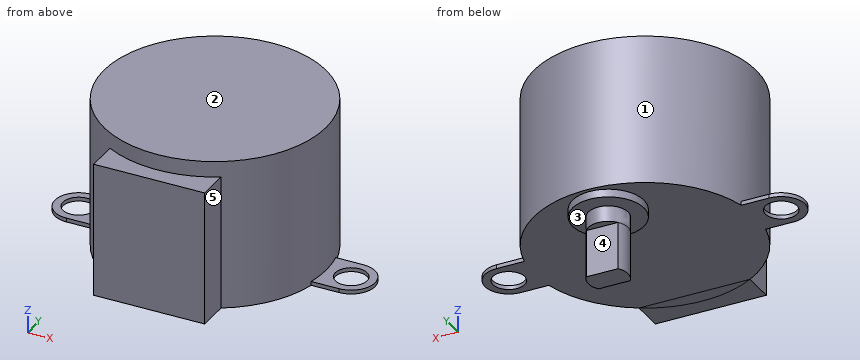
from build123d import *
from build123d.topology import SkipClean

# Parameters (mm, degrees)
SKETCH1_R           = 14
BOSS_EXTRUDE1_DEPTH = 19
SKETCH2_R           = 2
BOSS_EXTRUDE2_DEPTH = 0.5
SKETCH3_R           = 4.5
BOSS_EXTRUDE3_DEPTH = 1
SKETCH4_R           = 2.5
BOSS_EXTRUDE4_DEPTH = 2
BOSS_EXTRUDE5_DEPTH = 6
SKETCH6_W           = 14
SKETCH6_H           = 4
BOSS_EXTRUDE6_DEPTH = 17


with BuildPart() as part:
    # Sketch1 → Boss-Extrude1 (new body)
    with BuildSketch(Plane.XY):
        Circle(SKETCH1_R)
    extrude(amount=BOSS_EXTRUDE1_DEPTH)

    # Sketch2 → Boss-Extrude2 (add)
    # profile 1 of 2: a face of its own
    with BuildSketch(Plane(origin=(0, 0, 0), x_dir=(-1, 0, 0), z_dir=(0, 0, -1))):
        with BuildLine():
            Line((17.174794331, 3), (13.674794331, 3))
            ThreePointArc((13.674794331, 3), (14, 0), (13.674794331, -3))
            Line((13.674794331, -3), (17.174794331, -3))
            ThreePointArc((17.174794331, -3), (20.174794331, 0), (17.174794331, 3))
        make_face()
        with Locations((17.174794331, 0)):
            Circle(SKETCH2_R, mode=Mode.SUBTRACT)
    # profile 2 of 2: a face of its own
    with BuildSketch(Plane(origin=(0, 0, 0), x_dir=(-1, 0, 0), z_dir=(0, 0, -1))):
        with BuildLine():
            Line((-17.174794331, -3), (-13.674794331, -3))
            ThreePointArc((-13.674794331, -3), (-14, 0), (-13.674794331, 3))
            Line((-13.674794331, 3), (-17.174794331, 3))
            ThreePointArc((-17.174794331, 3), (-20.174794331, 0), (-17.174794331, -3))
        make_face()
        with Locations(Location((-17.174794331, 0, 0), (0, 0, 180))):
            Circle(SKETCH2_R, mode=Mode.SUBTRACT)
    extrude(amount=-BOSS_EXTRUDE2_DEPTH)

    # Sketch3 → Boss-Extrude3 (add)
    with BuildSketch(Plane(origin=(0, 0, 0), x_dir=(-1, 0, 0), z_dir=(0, 0, -1))):
        with Locations(Location((0, 9, 0), (0, 0, 180))):
            Circle(SKETCH3_R)
    extrude(amount=BOSS_EXTRUDE3_DEPTH)

    # Sketch4 → Boss-Extrude4 (add)
    with BuildSketch(Plane(origin=(0, 0, -1), x_dir=(-1, 0, 0), z_dir=(0, 0, -1))):
        with Locations((0, 9)):
            Circle(SKETCH4_R)
    extrude(amount=BOSS_EXTRUDE4_DEPTH)

    # Sketch5 → Boss-Extrude5 (add)
    with SkipClean():  # the faces are left unmerged after this step: merging them gives an invalid solid
        with BuildSketch(Plane(origin=(0, 0, -3), x_dir=(-1, 0, 0), z_dir=(0, 0, -1))):
            with BuildLine():
                Line((-2, 10.5), (2, 10.5))
                ThreePointArc((2, 10.5), (2.5, 9), (2, 7.5))
                Line((2, 7.5), (-2, 7.5))
                ThreePointArc((-2, 7.5), (-2.5, 9), (-2, 10.5))
            make_face()
        extrude(amount=BOSS_EXTRUDE5_DEPTH)

    # Sketch6 → Boss-Extrude6 (add)
    with SkipClean():  # the faces are left unmerged after this step: merging them gives an invalid solid
        with BuildSketch(Plane(origin=(0, 0, 0), x_dir=(-1, 0, 0), z_dir=(0, 0, -1))):
            with Locations((0, -14.124355653)):
                Rectangle(SKETCH6_W, SKETCH6_H)
        extrude(amount=-BOSS_EXTRUDE6_DEPTH)


solid = part.part
CAD build for the part. Positions are in the model's coordinates, mm. Face numbers are marked on the shaded views. A direction names the side the tool comes from. Round coordinates to 2 decimals unless told otherwise and drop trailing zeros. Loops run counter-clockwise (first coordinate to the right, second up) from the corner with the lowest first, then second, coordinate; pieces in that order, holes last.
(1) Which spindle directions (+Z, -Z, +X, -X, +Y, -Y) get a long thin tool onto all of the face, cutting with end or side? Do the marked faces 1, 2, 3, 4 and 5. Say none if no direction does.
(2) Cut at B-B (x = 0). Give the cut face in (y, z), plus the area to 3 significant figures.
(3) Drop flat-ended pins along their axis: pin 1 (8 mm diameter, centred on y = 2, z = 9, fed in from +X); pin 2 (6.5 mm diameter, centred on x = -17.17, y = 0, fed in from -Z); pin 3 (1.2 mm diameter, centred on x = 0, z = -7.5, fed in from +Y). Give the stop position or say it passes through.
(4) Cut at D-D (y = 8.5). Give the cut face in (x, z).
(5) Wall check: line 1 along Y through (x, z) = (-2, -2); line 2 along X through (y, z) = (-13.5, 11.5); line 3 along Z through (x, y) = (3, 0). Give the ranges that are in metal, low to high.
(6) Cut at A-A (y = 0). Give the cut face in (x, z), plus the area to 3 significant figures.
(7) Cut at C-C (z = 16). Give the cut face in (x, y), plus the area to 3 significant figures.
Findings below:
1. face 1: +Z
1. face 2: +Z, +X, -X, +Y, -Y
1. face 3: -Z
1. face 4: -Z, +X, -X, +Y
1. face 5: +Z, -Z, +X, -Y
2. outline: (-16.12, 0) - (4.5, 0) - (4.5, -1) - (6.5, -1) - (6.5, -3) - (7.5, -3) - (7.5, -9) - (10.5, -9) - (10.5, -3) - (11.5, -3) - (11.5, -1) - (13.5, -1) - (13.5, 0) - (14, 0) - (14, 19) - (-14, 19) - (-14, 17) - (-16.12, 17) - close
2. area: 605 mm2
3. pin 1: stops at x = 14
3. pin 2: stops at z = 0
3. pin 3: stops at y = 10.5
4. outline: (-11.12, 0) - (-4.47, 0) - (-4.47, -1) - (-2.45, -1) - (-2.45, -9) - (2.45, -9) - (2.45, -1) - (4.47, -1) - (4.47, 0) - (11.12, 0) - (11.12, 19) - (-11.12, 19) - close
5. line 1: y = 7.5 to 10.5
5. line 2: x = -7 to 7
5. line 3: z = 0 to 19
6. outline: (-20.17, 0) - (-19.17, 0) - (-19.17, 0.5) - (-20.17, 0.5) - close; (-15.17, 0) - (15.17, 0) - (15.17, 0.5) - (14, 0.5) - (14, 19) - (-14, 19) - (-14, 0.5) - (-15.17, 0.5) - close; (19.17, 0) - (20.17, 0) - (20.17, 0.5) - (19.17, 0.5) - close
6. area: 534 mm2
7. outline: (-7, -16.12) - (7, -16.12) - (7, -12.12) arc R14 ccw (long way) to (-7, -12.12) - close
7. area: 654 mm2
